Geometry check sheet. Reference: the model listing, model coordinates, mm. A direction names the side the tool comes from. Give positions to 0.01 mm unless a question says otherwise; leave off trailing zeros. Write each loop counter-clockwise with the first axis right and the second up, starting at its lowest first coordinate (ties: lowest second). Pieces come first, ordered by that corner, then holes. Notation, with made-up numbers: M 11,1.5 L 22,1.5 A11 cw 22,17.5 Z; hole C -28,36 d9. An arc over 180 degrees is marked long. One line per item, written item: value. Start each with the question number.
1. Tool access check on faces 5 (the face through (10, 0, 5)), 6 (the face through (-9.75, 0.05, 2.46)). Record the directions out of +Z, -Z, +X, -X, +Y, -Y that give a thin tool (end or side, any length) a straight path to the whole face; none if there is none.
2. Gauge pin test, flat ends, axial feed: pin 1 (8 mm diameter, centred on x = 0, y = 0, fed in from +Z); pin 2 (4 mm diameter, centred on x = -8.5, y = 0, fed in from +Z); pin 3 (2 mm diameter, centred on y = 9, z = 5, fed in from -X); pin 4 (1 mm diameter, centred on y = 6.5, z = 2.5, fed in from -X). Record the tip position at first contact, or that the pin passes through.
3. Scan lines: line 1 (Y direction, x = 0, z = 6.75); line 2 (X direction, y = -4.5, z = 2.5); line 3 (Y direction, x = -8.5, z = 2.15). Record each from-to range of solid material in increasing order.
4. Cross-section at C-C on z = 2.5. Record the cut outline in (x, y).
5. Cross-section at B-B on y = -0.5. Record the cut outline in (x, z), then the cut area to 3 significant figures.
6. Release check for a two-part mould opening along Y. For faces 1 (the face through (4, -4, 10)), 2 (the face through (4.619, -1.915, 4.93)), 3 (the face through (-4.336, -19.524, 4.93)), 4 (the face through (7.25, 0.05, 2.46)) record: pulls with the +Y half, pulls with the -Y half, needs draft (parallel to the pull), parting line crosses it, or undercut.
7. Cross-section at D-D on y = 16.5. Record the cut outline in (x, z), then the cut area to 3 significant figures.
8. Cross-section at A-A on x = 0. Record the cut outline in (y, z), then the cut area to 3 significant figures.
from build123d import *

# Parameters (mm, degrees)
SKETCH1_R           = 20
SKETCH1_R_2         = 1.25
SKETCH1_R_3         = 5
SKETCH1_R_4         = 1.5
BOSS_EXTRUDE1_DEPTH = 10
SKETCH2_R           = 4
CUT_EXTRUDE1_DEPTH  = 5


with BuildPart() as part:
    # Sketch1 → Boss-Extrude1 (new body)
    with BuildSketch(Plane.XY):
        Circle(SKETCH1_R)
        with Locations((-8.5, 0)):
            Circle(SKETCH1_R_2, mode=Mode.SUBTRACT)
        with Locations((8.5, 0)):
            Circle(SKETCH1_R_2, mode=Mode.SUBTRACT)
        Circle(SKETCH1_R_3, mode=Mode.SUBTRACT)
        with Locations((0, 16.5)):
            Circle(SKETCH1_R_4, mode=Mode.SUBTRACT)
        with Locations((0, -16.5)):
            Circle(SKETCH1_R_4, mode=Mode.SUBTRACT)
    extrude(amount=BOSS_EXTRUDE1_DEPTH)

    # Sketch2 → Cut-Extrude1 (cut)
    with BuildSketch(Plane.XY.offset(10)):
        with Locations((8.5, 0)):
            Circle(SKETCH2_R)
        with Locations((-8.5, 0)):
            Circle(SKETCH2_R)
    extrude(amount=-CUT_EXTRUDE1_DEPTH, mode=Mode.SUBTRACT)


solid = part.part
Report:
1. face 5: +Z
1. face 6: +Z, -Z
2. pin 1: passes through
2. pin 2: stops at z = 5
2. pin 3: stops at x = -18.33
2. pin 4: stops at x = -19.08
3. line 1: y = -20 to -18, -15 to -5, 5 to 15, 18 to 20
3. line 2: x = -19.49 to -2.18, 2.18 to 19.49
3. line 3: y = -18.1 to -1.25, 1.25 to 18.1
4. outline: C 0,0 d40; hole C -8.5,0 d2.5; hole C 0,0 d10; hole C 0,-16.5 d3; hole C 0,16.5 d3; hole C 8.5,0 d2.5
5. outline: M -19.99,0 L -9.65,0 L -9.65,5 L -12.47,5 L -12.47,10 L -19.99,10 Z; M -7.35,0 L -4.97,0 L -4.97,5 L -7.35,5 Z; M 4.97,0 L 7.35,0 L 7.35,5 L 4.97,5 Z; M 9.65,0 L 19.99,0 L 19.99,10 L 12.47,10 L 12.47,5 L 9.65,5 Z
5. area: 203 mm^2
6. face 1: needs draft
6. face 2: undercut
6. face 3: parting line crosses it
6. face 4: undercut
7. outline: M -11.3,0 L -1.5,0 L -1.5,10 L -11.3,10 Z; M 1.5,0 L 11.3,0 L 11.3,10 L 1.5,10 Z
7. area: 196 mm^2
8. outline: M -20,0 L -18,0 L -18,10 L -20,10 Z; M -15,0 L -5,0 L -5,10 L -15,10 Z; M 5,0 L 15,0 L 15,10 L 5,10 Z; M 18,0 L 20,0 L 20,10 L 18,10 Z
8. area: 240 mm^2
